```python
from build123d import *

# Parameters (mm, degrees)
F0_W           = 40.5
F0_H           = 20.5
F1_DEPTH       = 10
F2_SIZE        = 2
F3_R           = 2.9
F4_DEPTH       = 3
F7_DEPTH       = 126.422950013
F7_DEPTH_BACK  = 72.2858581577
F8_R           = 3
F9_R           = 1
F10_DEPTH      = 4
F12_DEPTH      = 3.596245468
F12_DEPTH_BACK = 3.8025450309
F13_R          = 1
F14_DEPTH      = 5.851831237
F15_R          = 1
F16_DEPTH      = 5
F17_R          = 1
F18_DEPTH      = 10.001
F18_DEPTH_BACK = 10.001


with BuildPart() as f1:
    # F0 (on Top) → F1 (new body, symmetric)
    with BuildSketch(Plane.XY):
        Polygon((7, 24.8), (-44.8, 24.8), (-44.8, -4.3), (0, -4.3), (19.0412067101, -13.3135236694), (86.5428958395, -176.8274940062), (92.1810515642, -174.7753731462), (36.5554890963, 0), align=None)
        with Locations((-20.25, 10.25)):
            Rectangle(F0_W, F0_H, mode=Mode.SUBTRACT)
        Polygon((6, -0.5019311232), (6, 18.0000764784), (27.0662221858, 0.3234172121), (18.3128683715, -6.3304656376), align=None, mode=Mode.SUBTRACT)
        Polygon((23.1584805053, -10.1837681409), (32.3305180335, -3.2116218642), (72.8933752329, -130.660014085), align=None, mode=Mode.SUBTRACT)
    extrude(amount=F1_DEPTH, both=True)

    # F2
    f2_edges = [f1.edges().sort_by_distance(p)[0] for p in [
        (-44.8, 24.8, 0),
        (-44.8, -4.3, 0),
    ]]
    chamfer(f2_edges, length=F2_SIZE)

    # F3 (on face) → F4 (join)
    with BuildSketch(Plane(origin=(0, 24.8, 0), x_dir=(-1, 0, 0), z_dir=(0, 1, 0))):
        with Locations((10.25, 0)):
            Circle(F3_R)
    extrude(amount=F4_DEPTH)

    # F6 (on mid) → F7 (cut, two sides)
    with BuildSketch(Plane(origin=(22.4071169072, 8.1555235899, 0), x_dir=(-0.3420201433, 0.9396926208, 0), z_dir=(0.9396926208, 0.3420201433, 0))) as f7_sk:
        Polygon((-35.7629049085, -10), (-195.7629049085, -3), (-195.7629049085, -10), align=None)
        Polygon((-35.7629049085, 10), (-195.7629049085, 10), (-195.7629049085, 3), align=None)
    extrude(amount=-F7_DEPTH, mode=Mode.SUBTRACT)
    extrude(f7_sk.sketch, amount=F7_DEPTH_BACK, mode=Mode.SUBTRACT)

    # F8
    f8_edges = [f1.edges().sort_by_distance(p)[0] for p in [
        (92.181052, -174.775373, 0),
        (89.361974, -175.801434, 3),
        (86.542896, -176.827494, 0),
        (89.361974, -175.801434, -3),
    ]]
    fillet(f8_edges, radius=F8_R)

    # F9 (on face) → F10 (cut)
    with BuildSketch(Plane(origin=(0, 24.8, 0), x_dir=(-1, 0, 0), z_dir=(0, 1, 0))):
        with Locations((15.25, 5)):
            Circle(F9_R)
        with Locations((15.25, -5)):
            Circle(F9_R)
        with Locations((5.25, -5)):
            Circle(F9_R)
        with Locations((5.25, 5)):
            Circle(F9_R)
    extrude(amount=-F10_DEPTH, mode=Mode.SUBTRACT)

    # F11 (on mid) → F12 (join, two sides)
    with BuildSketch(Plane(origin=(22.4071169072, 8.1555235899, 0), x_dir=(-0.3420201433, 0.9396926208, 0), z_dir=(0.9396926208, 0.3420201433, 0))) as f12_sk:
        Polygon((-59.0230961969, -8.9823666311), (-59.0230961969, 8.9823666311), (-65.0230961969, 8.7198666311), (-65.0230961969, -8.7198666311), align=None)
    extrude(amount=F12_DEPTH)
    extrude(f12_sk.sketch, amount=-F12_DEPTH_BACK)

    # F13 (on face) → F14 (cut, through all)
    with BuildSketch(Plane(origin=(15.1038475155, 18.0000645386, 0), x_dir=(-0.7660444431, 0.6427876097, 0), z_dir=(0.6427876097, 0.7660444431, 0))):
        with Locations((1.2878461653, 5)):
            Circle(F13_R)
        with Locations((1.2878461653, -5)):
            Circle(F13_R)
        with Locations((-18.7121538347, -5)):
            Circle(F13_R)
        with Locations((-18.7121538347, 5)):
            Circle(F13_R)
    extrude(amount=-F14_DEPTH, mode=Mode.SUBTRACT)

    # F15 (on face) → F16 (cut, through all)
    with BuildSketch(Plane(origin=(33.19318295, 10.5643572001, 0), x_dir=(-0.3032789919, 0.9529018066, 0), z_dir=(0.9529018066, 0.3032789919, 0))):
        with Locations((-24.0865118803, 0)):
            Circle(F15_R)
        with Locations((-44.0865118803, 0)):
            Circle(F15_R)
    extrude(amount=-F16_DEPTH, mode=Mode.SUBTRACT)

    # F17 (on Top) → F18 (cut, two sides)
    with BuildSketch(Plane.XY) as f18_sk:
        with Locations((84.231671552, -161.7060442644)):
            Circle(F17_R)
    extrude(amount=-F18_DEPTH, mode=Mode.SUBTRACT)
    extrude(f18_sk.sketch, amount=F18_DEPTH_BACK, mode=Mode.SUBTRACT)


solid = f1.part
```
Could you check a few things on this model? Use its own coordinates, in mm. A direction names the side the tool comes from. Round coordinates to 2 decimals unless told otherwise and drop trailing zeros. Loops run counter-clockwise (first coordinate to the right, second up) from the corner with the lowest first, then second, coordinate; pieces in that order, holes last. Notation, with made-up numbers: M -26.75,-27 L -3.75,-27 A29 cw -3.75,8 Z; hole C 65.5,12.5 d3. An arc over 180 degrees is marked long. Answer as CSV lines item,"result".
1) We'd pull the mould along X, two halves only. Please class faces 1 (the cylindrical face through (-7.353, 26.279, 0.128)), 2 (the cylindrical face through (13.03, 15.98, 5.04)), 3 (the flat face through (2, 2, -10)): released by +X, released by -X, zero draft, split by the parting line, or undercut.
From the geometry:
face 1,"split by the parting line"
face 2,"undercut"
face 3,"zero draft"
2) If I drill on probe 1 along Z at (x, y) = (-5, 22); probe 2 along X at (y, z) = (14.5, -6.5); probe 3 along Y at (x, z) = (-29, -0.5), over which ranges is the centre line in solid material (lowest first)?
From the geometry:
probe 1,"-10 to -5.97, -4.03 to 4.03, 5.97 to 10"
probe 2,"-44.8 to -40.5, 0 to 6, 10.17 to 19.28"
probe 3,"-4.3 to 0, 20.5 to 24.8"
3) Which directions (+Z, -Z, +X, -X, +Y, -Y) give clear straight access to the entire face, cutting with the end or side of a thin tool? Please do faces 4 (the flat face through (-21, 0, 0)), 5 (the flat face through (-22, -4.3, 0)), 6 (the flat face through (58.231, -68.105, 0.14)).
From the geometry:
face 4,"+Z, -Z"
face 5,"+Z, -Z, -X, -Y"
face 6,"+Z, -Z, +X, +Y"
4) Imagine slicing it at C-C on x = 69. List the corners of the cut face in (y, z) for me, and give its area (3 significant figures).
From the geometry:
outline,"M -134.33,-5.01 L -121.23,-5.55 L -121.23,5.55 L -134.33,5.01 Z; M -118.43,-5.66 L -101.94,-6.34 L -101.94,6.34 L -118.43,5.66 Z"
area,"336 mm^2"
5) For pin 1 Ø2 at (x, z) = (-15.5, 5) entering from +Y; pin 2 Ø1.5 at (x, z) = (37, 2) entering from -Y; pin 3 Ø10 at (x, z) = (17, -7.5) entering from +Y, each with a flat end and sliding along its axis, tell me the tip position at first contact or that it passes through.
From the geometry:
pin 1,"y = 24.8"
pin 2,"y = -58.63"
pin 3,"y = 20.6"
6) Imagine slicing it at B-B on y = -58. List the corners of the cut face in (x, z) for me, and give its area (3 significant figures).
From the geometry:
outline,"M 37.49,-8.62 L 42.9,-8.54 L 42.9,8.54 L 37.49,8.62 Z; M 49.77,-8.44 L 55.02,-8.36 L 55.02,8.36 L 49.77,8.44 Z"
area,"181 mm^2"
7) Imagine slicing it at A-A on x = -10.25. List the corners of the cut face in (y, z) for me, and give its area (3 significant figures).
From the geometry:
outline,"M -4.3,-10 L 0,-10 L 0,10 L -4.3,10 Z; M 20.5,-10 L 24.8,-10 L 24.8,-2.9 L 27.8,-2.9 L 27.8,2.9 L 24.8,2.9 L 24.8,10 L 20.5,10 Z"
area,"189 mm^2"
